Here's how the part is built. I have some questions about the finished solid (model axes, mm). A direction names the side the tool comes from. Coordinates: 2 decimals unless noted, no trailing zeros. Write each loop counter-clockwise with the first axis right and the second up, starting at its lowest first coordinate (ties: lowest second). Pieces come first, ordered by that corner, then holes.
Item 1: I want a section at A-A (z = 38.1). Please give me the cut outline in (x, y).
Item 2: If we mould it in two halves opening along Z, with no side actions, what happens to faces 1 (the face through (-82.55, 105.3, 6.44)), 2 (the face through (-5, -39.125, 41)), 3 (the face through (-5, -102, 76.2))? For each: pulls with the +Z half, pulls with the -Z half, needs draft (parallel to the pull), parting line crosses it, or undercut.
Item 3: For faces 4 (the face through (-11.355, -105, 44)), 5 (the face through (-106.588, 61, 25)), 6 (the face through (-4.917, -32.636, 21.297)), which set-ups out of +Z, -Z, +X, -X, +Y, -Y let a thin tool reach every point of the face, with its end or its side?
Item 4: Please list where these lines run through material, in increasing order: line 1 (Y direction, x = -103, z = 38); line 2 (Y direction, x = -9, z = 50); line 3 (X direction, y = 12, z = 44).
Item 5: I want a section at B-B (y = -68). Please give me the cut outline in (x, z).
Item 6: I want a section at C-C (z = 18). Please give me the cut outline in (x, y), and give its area (3 significant figures).
Item 7: I'm going to push flat-ended pins straight in: P1, Ø4, axis at x = -7, z = 45.5, coming from the +Y side; P2, Ø4, axis at x = -100, y = 77, coming from the +Z side; P3, Ø10, axis at x = -71.5, y = -63.5, coming from the +Z side; P4, Ø6, axis at x = -57, z = 17, coming from the -Y side. Where does each tip first touch, or does it pass through?
Item 8: I want a section at D-D (z = 72.5). Please give me the cut outline in (x, y).
from build123d import *

# Parameters (mm, degrees)
EXTRUDE1_DEPTH          = 12.7
SKETCH2_W               = 12.7
SKETCH2_H               = 127
EXTRUDE2_DEPTH          = 38.1
SKETCH3_W               = 12.7
SKETCH3_H               = 203.2
EXTRUDE3_DEPTH          = 63.5
F_1_2_20_TAPPED_HOLE1_D = 12.7
F_1_2_20_TAPPED_HOLE2_D = 12.7
CUT_EXTRUDE1_REACH      = 109.933


with BuildPart() as part:
    # Sketch1 → Extrude1 (new body)
    with BuildSketch(Plane.XY):
        Polygon((1.34455174, -204.860398808), (1.34455174, -1.660398808), (-11.35544826, -1.660398808), (-12.7, 0), (-71.443804275, 125.347638028), (-106.588300915, 125.347638028), (-106.588300915, -1.652361972), (-11.35544826, -204.860398808), align=None)
    extrude(amount=EXTRUDE1_DEPTH)

    # Sketch2 → Extrude2 (add)
    with BuildSketch(Plane.XY.offset(12.7)):
        with Locations((-100.238300915, 61.847638028)):
            Rectangle(SKETCH2_W, SKETCH2_H)
    extrude(amount=EXTRUDE2_DEPTH)

    # Sketch3 → Extrude3 (add)
    with BuildSketch(Plane.XY.offset(12.7)):
        with Locations((-5.00544826, -103.260398808)):
            Rectangle(SKETCH3_W, SKETCH3_H)
    extrude(amount=EXTRUDE3_DEPTH)

    # 1/2-20 Tapped Hole1 (through all)
    with Locations(Plane(origin=(-106.588300915, 99.947638028, 38.1), x_dir=(0, -1, 0), z_dir=(-1, 0, 0))):
        with Locations((0, 0)):
            Hole(F_1_2_20_TAPPED_HOLE1_D / 2)

    # 1/2-20 Tapped Hole2 (through all)
    with Locations(Plane(origin=(-85.963500915, 99.947638028, 0), x_dir=(-1, 0, 0), z_dir=(0, 0, -1))):
        with Locations((0, 0), (0, -50.8)):
            Hole(F_1_2_20_TAPPED_HOLE2_D / 2)

    # Sketch6 → Cut-Extrude1 (cut, up to next)
    with BuildSketch(Plane(origin=(1.34455174, 0, 0), x_dir=(0, 0, -1), z_dir=(1, 0, 0)), mode=Mode.PRIVATE) as cut_extrude1_sk1:
        with BuildLine():
            Line((-55.372, -26.425398808), (-27.645063582, -26.425398808))
            ThreePointArc((-27.645063582, -26.425398808), (-21.295063582, -32.775398808), (-27.645063582, -39.125398808))
            Line((-27.645063582, -39.125398808), (-55.372, -39.125398808))
            ThreePointArc((-55.372, -39.125398808), (-61.722, -32.775398808), (-55.372, -26.425398808))
        make_face()
    cut_extrude1_tool1 = extrude(cut_extrude1_sk1.sketch, amount=-CUT_EXTRUDE1_REACH, mode=Mode.PRIVATE) & part.part
    add(cut_extrude1_tool1.solids().sort_by_distance((1.344552, -32.775399, 41.508532))[0], mode=Mode.SUBTRACT)
    # Sketch6 → Cut-Extrude1 (cut, up to next)
    with BuildSketch(Plane(origin=(1.34455174, 0, 0), x_dir=(0, 0, -1), z_dir=(1, 0, 0)), mode=Mode.PRIVATE) as cut_extrude1_sk2:
        with BuildLine():
            Line((-55.372, -64.525398808), (-27.645063582, -64.525398808))
            ThreePointArc((-27.645063582, -64.525398808), (-21.295063582, -70.875398808), (-27.645063582, -77.225398808))
            Line((-27.645063582, -77.225398808), (-55.372, -77.225398808))
            ThreePointArc((-55.372, -77.225398808), (-61.722, -70.875398808), (-55.372, -64.525398808))
        make_face()
    cut_extrude1_tool2 = extrude(cut_extrude1_sk2.sketch, amount=-CUT_EXTRUDE1_REACH, mode=Mode.PRIVATE) & part.part
    add(cut_extrude1_tool2.solids().sort_by_distance((1.344552, -70.875399, 41.508532))[0], mode=Mode.SUBTRACT)
    # Sketch6 → Cut-Extrude1 (cut, up to next)
    with BuildSketch(Plane(origin=(1.34455174, 0, 0), x_dir=(0, 0, -1), z_dir=(1, 0, 0)), mode=Mode.PRIVATE) as cut_extrude1_sk3:
        with BuildLine():
            Line((-55.372, -110.245398808), (-27.645063582, -110.245398808))
            ThreePointArc((-27.645063582, -110.245398808), (-21.295063582, -116.595398808), (-27.645063582, -122.945398808))
            Line((-27.645063582, -122.945398808), (-55.372, -122.945398808))
            ThreePointArc((-55.372, -122.945398808), (-61.722, -116.595398808), (-55.372, -110.245398808))
        make_face()
    cut_extrude1_tool3 = extrude(cut_extrude1_sk3.sketch, amount=-CUT_EXTRUDE1_REACH, mode=Mode.PRIVATE) & part.part
    add(cut_extrude1_tool3.solids().sort_by_distance((1.344552, -116.595399, 41.508532))[0], mode=Mode.SUBTRACT)
    # Sketch6 → Cut-Extrude1 (cut, up to next)
    with BuildSketch(Plane(origin=(1.34455174, 0, 0), x_dir=(0, 0, -1), z_dir=(1, 0, 0)), mode=Mode.PRIVATE) as cut_extrude1_sk4:
        with BuildLine():
            Line((-55.372, -148.345398808), (-27.645063582, -148.345398808))
            ThreePointArc((-27.645063582, -148.345398808), (-21.295063582, -154.695398808), (-27.645063582, -161.045398808))
            Line((-27.645063582, -161.045398808), (-55.372, -161.045398808))
            ThreePointArc((-55.372, -161.045398808), (-61.722, -154.695398808), (-55.372, -148.345398808))
        make_face()
    cut_extrude1_tool4 = extrude(cut_extrude1_sk4.sketch, amount=-CUT_EXTRUDE1_REACH, mode=Mode.PRIVATE) & part.part
    add(cut_extrude1_tool4.solids().sort_by_distance((1.344552, -154.695399, 41.508532))[0], mode=Mode.SUBTRACT)


solid = part.part
Answer:
1. outline: (-106.59, -1.65) - (-93.89, -1.65) - (-93.89, 93.6) - (-106.59, 93.6) - close; (-106.59, 106.3) - (-93.89, 106.3) - (-93.89, 125.35) - (-106.59, 125.35) - close; (-11.36, -204.86) - (1.34, -204.86) - (1.34, -161.05) - (-11.36, -161.05) - close; (-11.36, -148.35) - (1.34, -148.35) - (1.34, -122.95) - (-11.36, -122.95) - close; (-11.36, -110.25) - (1.34, -110.25) - (1.34, -77.23) - (-11.36, -77.23) - close; (-11.36, -64.53) - (1.34, -64.53) - (1.34, -39.13) - (-11.36, -39.13) - close; (-11.36, -26.43) - (1.34, -26.43) - (1.34, -1.66) - (-11.36, -1.66) - close
2. face 1: needs draft
2. face 2: undercut
2. face 3: pulls with the +Z half
3. face 4: +Z, -X, +Y, -Y
3. face 5: +Z, -Z, -X, +Y, -Y
3. face 6: +X, -X
4. line 1: y = -1.65 to 93.6, 106.3 to 125.35
4. line 2: y = -204.86 to -161.05, -148.35 to -122.95, -110.25 to -77.23, -64.53 to -39.13, -26.43 to -1.66
4. line 3: x = -106.59 to -93.89
5. outline: (-75.49, 0) - (1.34, 0) - (1.34, 21.98) - (-11.36, 21.98) - (-11.36, 12.7) - (-75.49, 12.7) - close; (-11.36, 61.03) - (1.34, 61.03) - (1.34, 76.2) - (-11.36, 76.2) - close
6. outline: (-106.59, -1.65) - (-93.89, -1.65) - (-93.89, 125.35) - (-106.59, 125.35) - close; (-11.36, -204.86) - (1.34, -204.86) - (1.34, -1.66) - (-11.36, -1.66) - close
6. area: 4,190 mm2
7. P1: stops at y = -1.66
7. P2: stops at z = 50.8
7. P3: stops at z = 12.7
7. P4: passes through
8. outline: (-11.36, -204.86) - (1.34, -204.86) - (1.34, -1.66) - (-11.36, -1.66) - close
